Design review of the part built by this model. Coordinates are the model's own, in mm. Face numbers are marked on the shaded views. Coordinates: 2 decimals unless noted, no trailing zeros. Loops run counter-clockwise (first coordinate to the right, second up) from the corner with the lowest first, then second, coordinate; pieces in that order, holes last. Notation, with made-up numbers: (-32, -39.75) -> (-2, -39.75) arc R20 ccw to (-2, -22.75) -> close; hole circle Ø9 at (-35.5, 53). An arc over 180 degrees is marked (long way). Use a Markdown table: item, result. Add a question column.
Q1. Take a section at C-C on x = 61. Write out the cut boundary in (y, z), plus the area to 3 significant figures.
Q2. Draft analysis for pull direction Z (two halves, no side actions). For the marked faces 1 and 2, state which applies: pulls with the +Z half, pulls with the -Z half, needs draft (parallel to the pull), parting line crosses it, or undercut.
Q3. Clearance check with flat-ended pins moving along their axes: pin 1 Ø14 at (x, z) = (83, -17) entering from +Y; pin 2 Ø5 at (x, z) = (227.5, -35) entering from +Y. State where each tip first meets the part, or that it passes through.
Q4. Take a section at A-A on z = -3. Write out the cut boundary in (x, y).
Q5. For probe 1 along X at (y, z) = (-1.8, -3); probe 2 along X at (y, z) = (1.75, -22); probe 3 along Z at (x, y) = (130, 0.5), list the stretches that pass through material, from the lowest coordinate up.
Q6. Take a section at B-B on x = 3. Write out the cut boundary in (y, z).
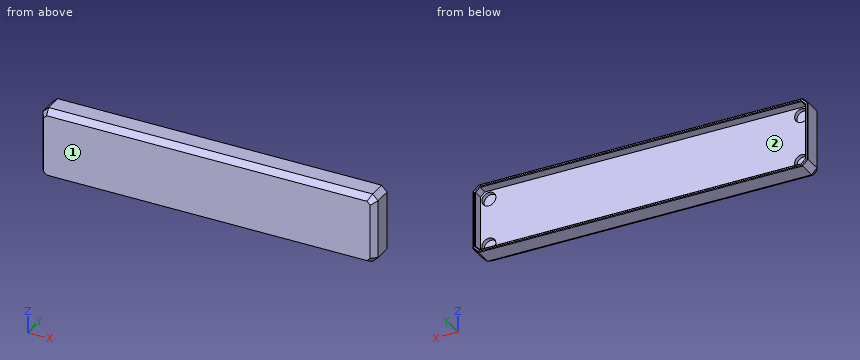
from build123d import *

# Parameters (mm, degrees)
SKETCH1_W           = 240
SKETCH1_H           = 50
BOSS_EXTRUDE1_DEPTH = 11
CHAMFER5_SIZE       = 4
SKETCH6_R           = 5
CUT_EXTRUDE5_DEPTH  = 3.1
CHAMFER9_SIZE       = 3
CHAMFER9_SIZE2      = 5.196152423
BOSS_EXTRUDE4_DEPTH = 7
CHAMFER13_SIZE      = 0.5
CHAMFER14_SIZE      = 0.5


with BuildPart() as part:
    # Sketch1 → Boss-Extrude1 (new body)
    with BuildSketch(Plane(origin=(0, 0, 0), x_dir=(1, 0, 0), z_dir=(0, 1, 0))):
        with Locations((115, 20)):
            Rectangle(SKETCH1_W, SKETCH1_H)
    extrude(amount=-BOSS_EXTRUDE1_DEPTH)

    # Chamfer5
    chamfer5_edges = [part.edges().sort_by_distance(p)[0] for p in [
        (-5, -5.5, 5),
        (-5, -5.5, -45),
        (235, -5.5, -45),
        (235, -5.5, 5),
    ]]
    chamfer(chamfer5_edges, length=CHAMFER5_SIZE)

    # Sketch6 → Cut-Extrude5 (cut)
    with BuildSketch(Plane(origin=(0, 0, 0), x_dir=(1, 0, 0), z_dir=(0, 1, 0))):
        with Locations(Location((3, 37, 0), (0, 0, 270))):
            Circle(SKETCH6_R)
        with Locations(Location((227, 37, 0), (0, 0, 270))):
            Circle(SKETCH6_R)
        with Locations(Location((227, 3, 0), (0, 0, 270))):
            Circle(SKETCH6_R)
        with Locations(Location((3, 3, 0), (0, 0, 270))):
            Circle(SKETCH6_R)
    extrude(amount=-CUT_EXTRUDE5_DEPTH, mode=Mode.SUBTRACT)

    # Chamfer9
    chamfer9_edges = [part.edges().sort_by_distance(p)[0] for p in [
        (115, -11, -45),
        (-5, -11, -20),
        (115, -11, 5),
        (235, -11, -20),
        (233, -11, -43),
        (233, -11, 3),
        (-3, -11, 3),
        (-3, -11, -43),
    ]]
    chamfer9_side = [part.faces().sort_by_distance(p)[0] for p in [
        (115, -11, -20),
    ]]
    chamfer(chamfer9_edges, length=CHAMFER9_SIZE, length2=CHAMFER9_SIZE2, reference=chamfer9_side[0])

    # Sketch8 → Boss-Extrude4 (add)
    with BuildSketch(Plane(origin=(0, 0, 0), x_dir=(1, 0, 0), z_dir=(0, 1, 0))):
        Polygon((-5, 41), (-1, 45), (231, 45), (235, 41), (235, -1), (231, -5), (-1, -5), (-5, -1), align=None)
        Polygon((-3.05, -0.05), (-0.05, -3.05), (230.05, -3.05), (233.05, -0.05), (233.05, 40.05), (230.05, 43.05), (-0.05, 43.05), (-3.05, 40.05), align=None, mode=Mode.SUBTRACT)
    extrude(amount=BOSS_EXTRUDE4_DEPTH)

    # Chamfer13
    chamfer13_edges = [part.edges().sort_by_distance(p)[0] for p in [
        (115, 7, 3.05),
        (231.55, 7, 1.55),
        (233.05, 7, -20),
        (231.55, 7, -41.55),
        (115, 7, -43.05),
        (-1.55, 7, -41.55),
        (-3.05, 7, -20),
        (-1.55, 7, 1.55),
    ]]
    chamfer(chamfer13_edges, length=CHAMFER13_SIZE)

    # Chamfer14
    chamfer14_edges = [part.edges().sort_by_distance(p)[0] for p in [
        (-5, 7, -20),
        (-3, 7, 3),
        (115, 7, 5),
        (233, 7, 3),
        (235, 7, -20),
        (233, 7, -43),
        (115, 7, -45),
        (-3, 7, -43),
    ]]
    chamfer(chamfer14_edges, length=CHAMFER14_SIZE)


solid = part.part
Answer list:
| question | item | result |
|---|---|---|
| 1 | outline | (-11, -42) -> (-5.8, -45) -> (6.5, -45) -> (7, -44.5) -> (7, -43.55) -> (6.5, -43.05) -> (0, -43.05) -> (0, 3.05) -> (6.5, 3.05) -> (7, 3.55) -> (7, 4.5) -> (6.5, 5) -> (-5.8, 5) -> (-11, 2) -> close |
| 1 | area | 561 mm² |
| 2 | face 1 | needs draft |
| 2 | face 2 | undercut |
| 3 | pin 1 | y = 0 |
| 3 | pin 2 | y = -3.1 |
| 4 | outline | (-5, -5.8) -> (-2, -11) -> (232, -11) -> (235, -5.8) -> (235, 6.5) -> (234.5, 7) -> (233.55, 7) -> (233.05, 6.5) -> (233.05, 0) -> (232, 0) -> (232, -3.1) -> (222, -3.1) -> (222, 0) -> (8, 0) -> (8, -3.1) -> (-2, -3.1) -> (-2, 0) -> (-3.05, 0) -> (-3.05, 6.5) -> (-3.55, 7) -> (-4.5, 7) -> (-5, 6.5) -> close |
| 5 | probe 1 | -5 to -2, 8 to 222, 232 to 235 |
| 5 | probe 2 | -5 to -3.05, 233.05 to 235 |
| 5 | probe 3 | -45 to -43.05, 3.05 to 5 |
| 6 | outline | (-11, -42) -> (-5.8, -45) -> (6.5, -45) -> (7, -44.5) -> (7, -43.55) -> (6.5, -43.05) -> (0, -43.05) -> (0, -42) -> (-3.1, -42) -> (-3.1, -32) -> (0, -32) -> (0, -8) -> (-3.1, -8) -> (-3.1, 2) -> (0, 2) -> (0, 3.05) -> (6.5, 3.05) -> (7, 3.55) -> (7, 4.5) -> (6.5, 5) -> (-5.8, 5) -> (-11, 2) -> close |
